Check sheet for the drawn part. Datum: minimum x, y, z corner. Units: mm. Round coordinates to 2 decimals unless told otherwise and drop trailing zeros. Write each loop counter-clockwise with the first axis right and the second up, starting at its lowest first coordinate (ties: lowest second). Pieces come first, ordered by that corner, then holes. Notation, with made-up numbers: M -36.75,86 L 12.25,86 A28 cw 12.25,108 Z; hole C 43.25,21 d11. An arc over 180 degrees is marked long. One line per item, written item: value.
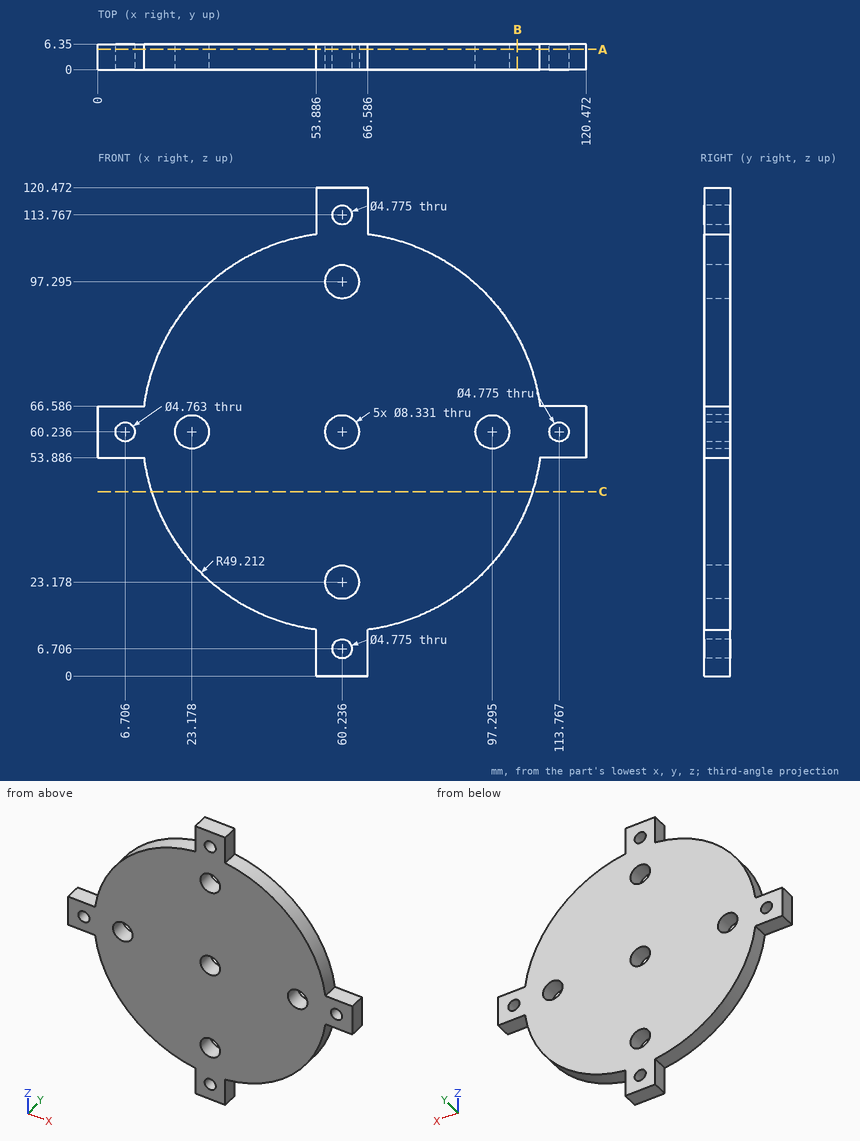
Q1. Sectioned sample at C-C on z = 45.5. Enter the section's corners in (x, y).
Completed:
outline: M 13.28,0 L 107.19,0 L 107.19,6.35 L 13.28,6.35 Z
Q2. Scan lines: line 1 (Z direction, x = 6.5, y = 4.5) (1 decimal); line 2 (Z direction, x = 27, y = 1) (1 decimal); line 3 (X direction, y = 4.75, z = 115) (1 decimal). Record each from-to range of solid material in increasing order. Write a range as [from, to].
Completed:
line 1: [53.9, 57.9], [62.6, 66.6]
line 2: [23.9, 58.6], [61.9, 96.5]
line 3: [53.9, 58.2], [62.3, 66.6]
Q3. Sectioned sample at B-B on x = 103.5. Enter the section's corners in (y, z).
Completed:
outline: M 0,36.78 L 6.35,36.78 L 6.35,83.69 L 0,83.69 Z
Q4. Depth check by flat-ended pin: P1, Ø1, axis at y = 4, z = 90, coming from the -X side; P2, Ø3, axis at x = 49, y = 3.5, coming from the -Z side; P3, Ø3, axis at y = 2.5, z = 20.5, coming from the +X side. Enter the tip coordinate at first touch or a pass-through.
Completed:
P1: x = 20.67
P2: z = 12
P3: x = 91.22
Q5. Sectioned sample at A-A on y = 5. State how many separate pieces and enclosed holes the cut face has, and give its area (3 significant figures).
Completed:
separate pieces: 1
enclosed holes: 9
area: 7,830 mm^2
